Input: dimensioned drawing with shaded views. Units: mm. Origin: part minimum x, y, z. A direction names the side the tool comes from. Give positions to 0.01 mm unless a question says otherwise; leave off trailing zeros. Write each loop counter-clockwise with the first axis right and the second up, starting at its lowest first coordinate (ties: lowest second). Pieces come first, ordered by that corner, then holes. Notation, with made-up numbers: (9, 48) -> (15, 48) arc R26 cw to (15, 79) -> close; hole circle Ø5 at (28.25, -34.75). An arc over 180 degrees is marked (long way). Answer as a JSON object with one key per item and string values.
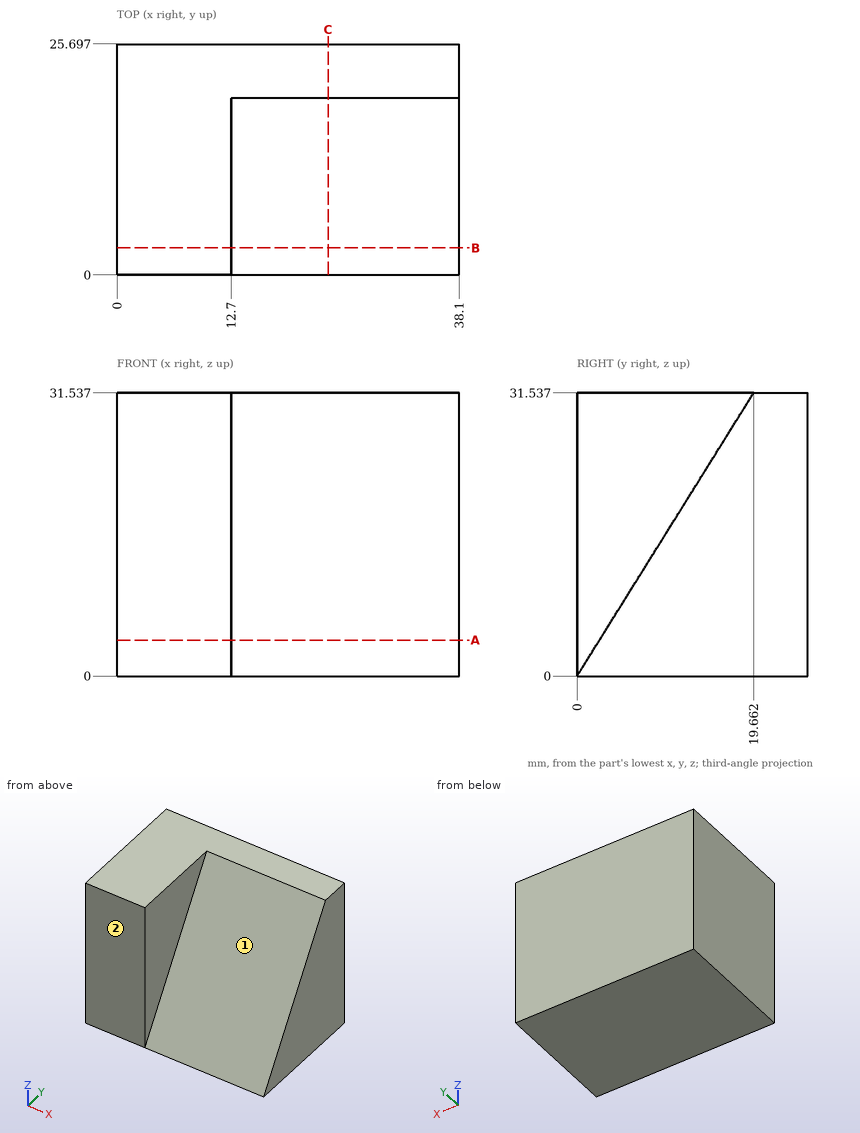
Q1. First-contact query: P1, Ø3, axis at x = 27.5, y = 5.5, coming from the +Z side; P2, Ø2, axis at x = 15.5, z = 20.5, coming from the -Y side. Flat tips, straight axial feed; report the tip coordinate or a pass-through.
Values:
{"P1": "z = 11.23", "P2": "y = 12.16"}
Q2. Material intervals for L1, parallel to X at y = 5.75, z = 22; L2, parallel to Y at x = 30, z = 3.5; L3, parallel to Y at x = 26.5, z = 29, sorted ascending. Write a range as from..to.
Values:
{"L1": "0..12.7", "L2": "2.18..25.7", "L3": "18.08..25.7"}
Q3. Cut plane B-B (y = 3). Return the cut outline in (x, z), and give its area (3 significant figures).
Values:
{"outline": "(0, 0) -> (38.1, 0) -> (38.1, 4.81) -> (12.7, 4.81) -> (12.7, 31.54) -> (0, 31.54) -> close", "area": "523 mm²"}
Q4. Cut plane A-A (z = 4). Return the cut outline in (x, y), and give its area (3 significant figures).
Values:
{"outline": "(0, 0) -> (12.7, 0) -> (12.7, 2.49) -> (38.1, 2.49) -> (38.1, 25.7) -> (0, 25.7) -> close", "area": "916 mm²"}
Q5. Set-up query: the marked faces 1 and 2. Return all of +Z, -Z, +X, -X, +Y, -Y with unobstructed straight access to the full face (end or side cutting, diameter ignored); none if empty.
Values:
{"face 1": "+Z, +X, -Y", "face 2": "+Z, -Z, +X, -X, -Y"}
Q6. Cut plane C-C (x = 23.5). Return the cut outline in (y, z).
Values:
{"outline": "(0, 0) -> (25.7, 0) -> (25.7, 31.54) -> (19.66, 31.54) -> close"}
